```python
from build123d import *

# Parameters (mm, degrees)
BOSS_EXTRUDE1_DEPTH = 5
SKETCH2_R           = 5
BOSS_EXTRUDE2_DEPTH = 12.5
SKETCH3_R           = 3.175
BOSS_EXTRUDE3_DEPTH = 50.8


with BuildPart() as part:
    # Sketch1 → Boss-Extrude1 (new, symmetric)
    with BuildSketch(Plane(origin=(0, 0, 0), x_dir=(1, 0, 0), z_dir=(0, 1, 0))):
        Polygon((5, 5), (-5, 5), (-5, 0), (-13.75, 0), (-13.75, -7.5), (-3.75, -7.5), (-3.75, -2.5), (3.75, -2.5), (3.75, -7.5), (13.75, -7.5), (13.75, 0), (5, 0), align=None)
    extrude(amount=BOSS_EXTRUDE1_DEPTH, both=True)

    # Sketch2 → Boss-Extrude2 (add)
    with BuildSketch(Plane(origin=(0, 0, -5), x_dir=(-1, 0, 0), z_dir=(0, 0, -1))):
        Circle(SKETCH2_R)
    extrude(amount=BOSS_EXTRUDE2_DEPTH)

    # Sketch3 → Boss-Extrude3 (add)
    with BuildSketch(Plane(origin=(0, 0, -17.5), x_dir=(-1, 0, 0), z_dir=(0, 0, -1))):
        Circle(SKETCH3_R)
    extrude(amount=BOSS_EXTRUDE3_DEPTH)


solid = part.part
```
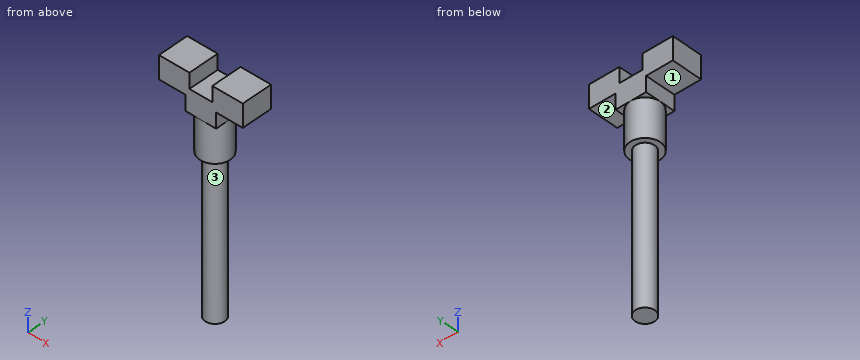
Could you check a few things on this model? Use its own coordinates, in mm. Face numbers are marked on the shaded views. A direction names the side the tool comes from. Give positions to 0.01 mm unless a question says otherwise; leave off trailing zeros. Order: outer loops, then holes, each group sorted by start corner. A loop starts at its lowest first (then second) coordinate and runs counter-clockwise, first axis right, second up.
Q1. If I drill on line 1 along X through (y, z) = (-4.5, 4); line 2 along Z through (x, y) = (-2.25, 2.75); line 3 along Z through (x, y) = (-4.75, 0.5), over which ranges is the centre line in solid material (lowest first)?
Q2. Suppose I cut it at B-B, the plane z = -11. Write out the boundary of the cut face in (x, y).
Q3. Suppose I cut it at A-A, the plane y = 2. Write out the boundary of the cut face in (x, z).
Q4. Suppose I cut it at C-C, the plane x = -2.5. Write out the boundary of the cut face in (y, z), and give its area (3 significant figures).
Q5. I'm going to push flat-ended pins straight in: P1, Ø2, axis at x = -3.5, y = -3, coming from the +Z side; P2, Ø12, axis at x = -10, z = -10.5, coming from the -Y side; P3, Ø1.5, axis at x = 3, y = -3.5, coming from the -Z side; P4, Ø4.5, axis at x = 11.5, y = 2, coming from the -Z side. Where does each tip first touch, or does it pass through?
Q6. Suppose I cut it at D-D, the plane y = -1. Write out the boundary of the cut face in (x, z), and give its area (3 significant figures).
Q7. For the marked faces 1, 2 and 3, which set-ups out of +Z, -Z, +X, -X, +Y, -Y let a thin tool reach every point of the face, with its end or its side?
Solution:
1. line 1: x = -13.75 to -3.75, 3.75 to 13.75
1. line 2: z = -17.5 to 2.5
1. line 3: z = -17.5 to 7.5
2. outline: circle Ø10 at (0, 0)
3. outline: (-13.75, 0) - (-5, 0) - (-5, -5) - (-4.58, -5) - (-4.58, -17.5) - (-2.47, -17.5) - (-2.47, -68.3) - (2.47, -68.3) - (2.47, -17.5) - (4.58, -17.5) - (4.58, -5) - (5, -5) - (5, 0) - (13.75, 0) - (13.75, 7.5) - (3.75, 7.5) - (3.75, 2.5) - (-3.75, 2.5) - (-3.75, 7.5) - (-13.75, 7.5) - close
4. outline: (-5, -5) - (-4.33, -5) - (-4.33, -17.5) - (-1.96, -17.5) - (-1.96, -68.3) - (1.96, -68.3) - (1.96, -17.5) - (4.33, -17.5) - (4.33, -5) - (5, -5) - (5, 2.5) - (-5, 2.5) - close
4. area: 382 mm2
5. P1: stops at z = 7.5
5. P2: stops at y = -3
5. P3: stops at z = -17.5
5. P4: stops at z = 0
6. outline: (-13.75, 0) - (-5, 0) - (-5, -5) - (-4.9, -5) - (-4.9, -17.5) - (-3.01, -17.5) - (-3.01, -68.3) - (3.01, -68.3) - (3.01, -17.5) - (4.9, -17.5) - (4.9, -5) - (5, -5) - (5, 0) - (13.75, 0) - (13.75, 7.5) - (3.75, 7.5) - (3.75, 2.5) - (-3.75, 2.5) - (-3.75, 7.5) - (-13.75, 7.5) - close
6. area: 647 mm2
7. face 1: -Z, -X, +Y, -Y
7. face 2: -Z, +X, +Y, -Y
7. face 3: -Z
